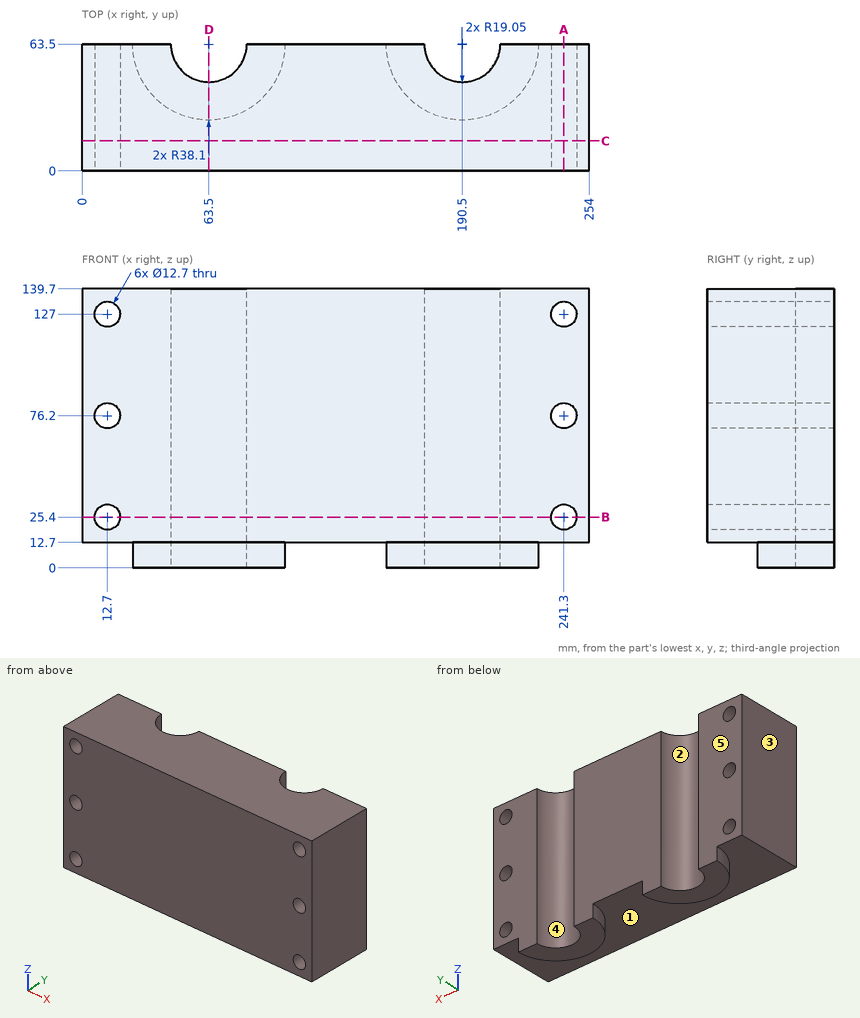
Input: dimensioned drawing with shaded views. Units: mm. Origin: part minimum x, y, z. A direction names the side the tool comes from. Give positions to 0.01 mm unless a question says otherwise; leave off trailing zeros. Write each loop counter-clockwise with the first axis right and the second up, starting at its lowest first coordinate (ties: lowest second). Pieces come first, ordered by that corner, then holes.
1. Section query A-A, the plane x = 241.3. Return loops of the section in (y, z), then the cut area to 3 significant figures.
2. Pin query (flat end, axial travel): P1, Ø7.5, axis at x = 241.3, z = 127, coming from the +Y side. Return the tip coordinate at first contact, or that it passes through.
3. Section query B-B, the plane z = 25.4. Return loops of the section in (x, y).
4. Draft query along X for the marked faces 3, 4 and 5. Return one class per face: released by +X, released by -X, zero draft, split by the parting line, or undercut.
5. Section query D-D, the plane x = 63.5. Return loops of the section in (y, z), then the cut area to 3 significant figures.
6. Reachability of the marked faces 1 and 2 from +Z, -Z, +X, -X, +Y, -Y: full face, straight path, thin tool, end or side. Return the list, or none.
7. Section query C-C, the plane y = 15. Return loops of the section in (x, z), then the cut area to 3 significant figures.
8. Line query: probe 1 along Z at (x, y) = (12, 48); probe 2 along X at (y, z) = (41.5, 127); probe 3 along X at (y, z) = (46, 76). Output: solid intervals per line, ascending.
Computed:
1. outline: (0, 12.7) - (63.5, 12.7) - (63.5, 19.05) - (0, 19.05) - close; (0, 31.75) - (63.5, 31.75) - (63.5, 69.85) - (0, 69.85) - close; (0, 82.55) - (63.5, 82.55) - (63.5, 120.65) - (0, 120.65) - close; (0, 133.35) - (63.5, 133.35) - (63.5, 139.7) - (0, 139.7) - close
1. area: 5,650 mm2
2. P1: passes through
3. outline: (0, 0) - (6.35, 0) - (6.35, 63.5) - (0, 63.5) - close; (19.05, 0) - (234.95, 0) - (234.95, 63.5) - (209.55, 63.5) arc R19.05 cw to (171.45, 63.5) - (82.55, 63.5) arc R19.05 cw to (44.45, 63.5) - (19.05, 63.5) - close; (247.65, 0) - (254, 0) - (254, 63.5) - (247.65, 63.5) - close
4. face 3: released by -X
4. face 4: undercut
4. face 5: zero draft
5. outline: (0, 12.7) - (25.4, 12.7) - (25.4, 0) - (44.45, 0) - (44.45, 139.7) - (0, 139.7) - close
5. area: 5,890 mm2
6. face 1: -Z, -Y
6. face 2: +Z, -Z, +Y
7. outline: (0, 12.7) - (254, 12.7) - (254, 139.7) - (0, 139.7) - close; hole circle Ø12.7 at (12.7, 25.4); hole circle Ø12.7 at (12.7, 76.2); hole circle Ø12.7 at (12.7, 127); hole circle Ø12.7 at (241.3, 25.4); hole circle Ø12.7 at (241.3, 76.2); hole circle Ø12.7 at (241.3, 127)
7. area: 31,500 mm2
8. probe 1: z = 12.7 to 19.09, 31.71 to 69.89, 82.51 to 120.69, 133.31 to 139.7
8. probe 2: x = 0 to 6.35, 19.05 to 234.95, 247.65 to 254
8. probe 3: x = 0 to 6.35, 19.05 to 55.97, 71.03 to 182.97, 198.03 to 234.95, 247.65 to 254
